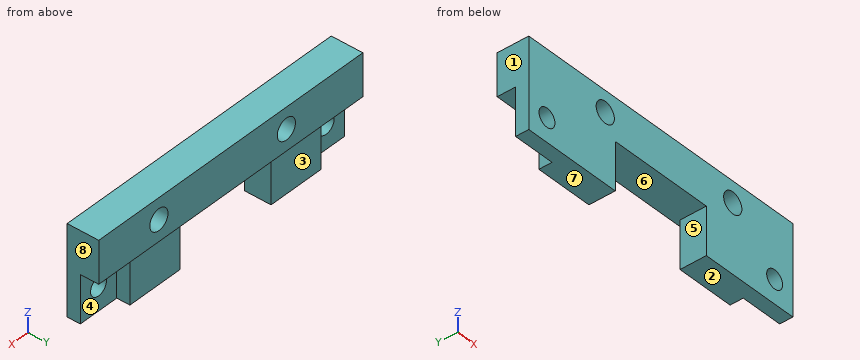
from build123d import *

# Parameters (mm, degrees)
F0_R     = 2
F0_W     = 8
F0_H     = 9
F0_R_2   = 1.75
F0_W_2   = 11
F1_DEPTH = 2.5
F2_DEPTH = 2.5
F3_DEPTH = 3.5


with BuildPart() as f1:
    # F0 (on Front) → F1 (new body)
    with BuildSketch(Plane.XZ):
        Polygon((-62.011425, 28.630727), (-62.011425, 20.630727), (-54.011425, 20.630727), (-43.011425, 20.630727), (-23.011425, 20.630727), (-12.011425, 20.630727), (-4.011425, 20.630727), (-4.011425, 28.630727), align=None)
        with Locations((-45.215137, 24.630727)):
            Circle(F0_R, mode=Mode.SUBTRACT)
        with Locations((-17.215137, 24.630727)):
            Circle(F0_R, mode=Mode.SUBTRACT)
        with Locations((-58.011425, 16.130727)):
            Rectangle(F0_W, F0_H)
        with Locations((-58.011425, 16.130727)):
            Circle(F0_R_2, mode=Mode.SUBTRACT)
        with Locations((-48.511425, 16.130727)):
            Rectangle(F0_W_2, F0_H)
        with Locations((-17.511425, 16.130727)):
            Rectangle(F0_W_2, F0_H)
        with Locations((-8.011425, 16.130727)):
            Rectangle(F0_W, F0_H)
        with Locations((-8.011425, 16.130727)):
            Circle(F0_R_2, mode=Mode.SUBTRACT)
    extrude(amount=F1_DEPTH)

    # F0 (on Front) → F2 (join)
    with BuildSketch(Plane.XZ):
        with Locations((-48.511425, 16.130727)):
            Rectangle(F0_W_2, F0_H)
        with Locations((-17.511425, 16.130727)):
            Rectangle(F0_W_2, F0_H)
    extrude(amount=-F2_DEPTH)

    # F0 (on Front) → F3 (join)
    with BuildSketch(Plane.XZ):
        Polygon((-62.011425, 28.630727), (-62.011425, 20.630727), (-54.011425, 20.630727), (-43.011425, 20.630727), (-23.011425, 20.630727), (-12.011425, 20.630727), (-4.011425, 20.630727), (-4.011425, 28.630727), align=None)
        with Locations((-45.215137, 24.630727)):
            Circle(F0_R, mode=Mode.SUBTRACT)
        with Locations((-17.215137, 24.630727)):
            Circle(F0_R, mode=Mode.SUBTRACT)
    extrude(amount=-F3_DEPTH)


solid = f1.part
Input: part model. Units: mm. Frame: model coordinates. Face numbers are marked on the shaded views. A direction names the side the tool comes from. Coordinates: 2 decimals unless noted, no trailing zeros. Order: outer loops, then holes, each group sorted by start corner. A loop starts at its lowest first (then second) coordinate and runs counter-clockwise, first axis right, second up. Notation, with made-up numbers: M 21.25,78 L 55.25,78 A18 cw 55.25,98 Z; hole C 3,-6 d3. An arc over 180 degrees is marked long. One line per question, with ' | ' between items.
Item 1: Section C-C (x = -7.5). Output: boundary loops of the cut face in (y, z), then the cut area to 3 significant figures.
Geometry results:
outline: M -2.5,11.63 L 0,11.63 L 0,14.46 L -2.5,14.46 Z; M -2.5,17.8 L 0,17.8 L 0,20.63 L 3.5,20.63 L 3.5,28.63 L -2.5,28.63 Z | area: 62.1 mm^2
Item 2: Reachability of the marked faces 1, 2, 3, 4 and 5 from +Z, -Z, +X, -X, +Y, -Y: full face, straight path, thin tool, end or side. Return the list, or none.
Geometry results:
face 1: +Z, -Z, -X, +Y, -Y | face 2: -Z, +X, -X, +Y, -Y | face 3: -Z, +X, -X, +Y | face 4: -Z, +X, +Y | face 5: -Z, +Y, -Y
Item 3: Ray query, line 1 along X through (y, z) = (-0.4, 24.75); line 2 along X through (y, z) = (0.4, 13); line 3 along X through (y, z) = (-0.75, 19). Return the intervals inside material, ascending.
Geometry results:
line 1: x = -62.01 to -47.21, -43.22 to -19.21, -15.22 to -4.01 | line 2: x = -54.01 to -43.01, -23.01 to -12.01 | line 3: x = -62.01 to -43.01, -23.01 to -4.01
Item 4: Draft query along X for the marked faces 6, 7 and 8. Return one class per face: released by +X, released by -X, zero draft, split by the parting line, or undercut.
Geometry results:
face 6: undercut | face 7: zero draft | face 8: released by +X
Item 5: Pin query (flat end, axial travel): pin 1 (6.5 mm diameter, centred on x = -17.22, z = 24.63, fed in from +Y); pin 2 (3 mm diameter, centred on x = -45.22, z = 24.63, fed in from -Y); pin 3 (2 mm diameter, centred on y = 1.5, z = 18, fed in from +X); pin 4 (4.5 mm diameter, centred on x = -17.5, z = 18, fed in from +Y). Return the tip coordinate at first contact, or that it passes through.
Geometry results:
pin 1: stops at y = 3.5 | pin 2: passes through | pin 3: stops at x = -12.01 | pin 4: stops at y = 2.5
Item 6: Section A-A (z = 13.5). Output: boundary loops of the cut face in (x, y), then the cut area to 3 significant figures.
Geometry results:
outline: M -62.01,-2.5 L -43.01,-2.5 L -43.01,2.5 L -54.01,2.5 L -54.01,0 L -62.01,0 Z; M -23.01,-2.5 L -4.01,-2.5 L -4.01,0 L -12.01,0 L -12.01,2.5 L -23.01,2.5 Z | area: 150 mm^2
Item 7: Section D-D (y = 1.7). Output: boundary loops of the cut face in (x, z), then the cut area to 3 significant figures.
Geometry results:
outline: M -62.01,20.63 L -54.01,20.63 L -54.01,11.63 L -43.01,11.63 L -43.01,20.63 L -23.01,20.63 L -23.01,11.63 L -12.01,11.63 L -12.01,20.63 L -4.01,20.63 L -4.01,28.63 L -62.01,28.63 Z; hole C -45.22,24.63 d4; hole C -17.22,24.63 d4 | area: 637 mm^2
Item 8: Section B-B (x = -49). Output: boundary loops of the cut face in (y, z).
Geometry results:
outline: M -2.5,11.63 L 2.5,11.63 L 2.5,20.63 L 3.5,20.63 L 3.5,28.63 L -2.5,28.63 Z
